Autodesk Inventor part; units mm, degrees
ref_plane "Work Plane5" through (-6.2, 0, 0) normal (-1, 0, 0) x (0, 0, 1)
ref_plane "YZ Plane" through (0, 0, 0) normal (1, 0, 0) x (0, 1, 0)
ref_plane "XZ Plane" through (0, 0, 0) normal (0, 1, 0) x (-1, 0, 0)
sketch "Sketch1" plane through (0, 0, 0) normal (0, 0, 1) x (1, 0, 0)
  line L0 (0, 0) -> (31, 0)
  line L1 (31, 0) -> (31, 4)
  line L2 (31, 4) -> (0, 4)
  line L3 (0, 4) -> (0, 0)
  line L4 (0, 18) -> (31, 18)
  line L5 (31, 18) -> (31, 20)
  line L6 (31, 20) -> (0, 20)
  line L7 (0, 20) -> (0, 18)
  line L8 (0, 34) -> (31, 34)
  line L9 (31, 34) -> (31, 38)
  line L10 (31, 38) -> (0, 38)
  line L11 (0, 38) -> (0, 34)
  line L12 (-7, 38) -> (0, 38)
  line L13 (0, 38) -> (0, 0)
  line L14 (0, 0) -> (-7, 0)
  line L15 (-7, 0) -> (-7, 38)
  line L16 (35, 38) -> (31, 38)
  line L17 (31, 38) -> (31, 0)
  line L18 (31, 0) -> (35, 0)
  line L19 (35, 0) -> (35, 38)
  point P0 (0, 4)
  point P1 (0, 18)
  point P2 (0, 20)
  point P3 (0, 34)
  dimension "d1" = 31
  dimension "d3" = 14
  dimension "d4" = 14
  dimension "d7" = 4
  dimension "d25" = 2
  dimension "d26" = 7
  dimension "d27" = 4
extrude "Extrusion1" add sketch "Sketch1" along normal blind 75 contours L3 L2 L1 L0 | L14 L15 L12 L11 L13 L7 L3 | L1 L17 L5 L9 L16 L19 L18 | L7 L6 L5 L4 | L10 L9 L8 L11
ref_plane "Work Plane5" through (-6.2, 0, 0) normal (-1, 0, 0) x (0, 0, 1)
sketch "Sketch4" plane through (-7, 0, 0) normal (-1, 0, 0) x (0, 0, 1)
  circle A0 centre (19, 19) radius 16.002
  circle A1 centre (56, 19) radius 16.002
  line L0 (75, 38) -> (75, 0)
  line L1 (0, 38) -> (0, 0)
  line L2 (56, 35.002) -> (72.002, 35.002)
  line L3 (72.002, 35.002) -> (72.002, 2.998)
  line L4 (72.002, 2.998) -> (56, 2.998)
  line L5 (19, 35.002) -> (35.002, 35.002)
  line L6 (35.002, 35.002) -> (35.002, 2.998)
  line L7 (35.002, 2.998) -> (19, 2.998)
  point P0 (0, 19)
  point P1 (35.002, 19)
  point P2 (72.002, 19)
  dimension "d28" = 32.004
  dimension "d29" = 32.004
  dimension "d32" = 19
  dimension "d33" = 19
extrude "Extrusion4" cut sketch "Sketch4" against normal blind 5.08 from surface at -0.8
fillet "Fillet2" radius 4 4 edges at (-7, 38, 37.5) (35, 38, 37.5) (35, 0, 37.5) (-7, 0, 37.5)
equation "\"d3\" = d4"
properties part number "Electronics Mount"
Read the model definition and answer for the solid it produces. Units are mm, in the model's axes. A direction names the side the tool comes from. Give positions to 0.01 mm unless a question says otherwise; leave off trailing zeros. Write each loop counter-clockwise with the first axis right and the second up, starting at its lowest first coordinate (ties: lowest second). Pieces come first, ordered by that corner, then holes. Notation, with made-up numbers: M 11,60 L 60,60 A25 cw 60,73 Z; hole C -33.5,-35.75 d2. An arc over 180 degrees is marked long. One line per item, written item: value. Start each with the question number.
(1) A tool of negligible diameter and unlimited length cuts with its end or side. For faces 1 (the flat face through (16, 4, 37)), 2 (the flat face through (-6.2, 19, 19)), 3 (the flat face through (14, 19, 75)), from which of +Z, -Z, +X, -X, +Y, -Y can it reach the whole face along a straight path? Write none if from no direction.
(2) Find section C-C (z = 20). Determine the outline of the cut face in (x, y), plus the area to 3 significant figures.
(3) Determine the mould class of faces 4 (the flat face through (-4, 19, 35.002)), 5 (the flat face through (-4, 35.002, 27)), 6 (the flat face through (14, 19, 0)), 7 (the cylindrical face through (-5.859, 1.203, 38.025)) for opening direction X: pulls with the +X half, pulls with the -X half, needs draft (parallel to the pull), parting line crosses it, or undercut.
(4) Flat-ended cylindrical pins translate along their axes: pin 1 Ø1.5 at (x, z) = (-5, 63) entering from -Y; pin 2 Ø1.5 at (x, z) = (-4, 26) entering from -Y. Find the tip coordinate at first contact, or state that the pin passes through.
(5) Find section A-A (x = 12). Determine the outline of the cut face in (y, z), plus the area to 3 significant figures.
(6) Find the intervals of material crossed by line 1 (X direction, y = 10, z = 14); line 2 (Y direction, x = 29, z = 45.5); line 3 (Z direction, x = -3, y = 23.5), in increasing order.
(7) Find section B-B (y = 7). Determine the outline of the cut face in (x, z).
(8) Find section D-D (y = 19). Determine the outline of the cut face in (x, z), plus the area to 3 significant figures.
Results below:
1. face 1: +Z, -Z
1. face 2: none
1. face 3: +Z, +X, -X, +Y, -Y
2. outline: M -7,4 A4 ccw -3,0 L 31,0 A4 ccw 35,4 L 35,34 A4 ccw 31,38 L -3,38 A4 ccw -7,34 Z; hole M -6.2,3 L -1.12,3 L -1.12,35 L -6.2,35 Z; hole M 0,4 L 31,4 L 31,18 L 0,18 Z; hole M 0,20 L 31,20 L 31,34 L 0,34 Z
2. area: 552 mm^2
3. face 4: undercut
3. face 5: undercut
3. face 6: needs draft
3. face 7: pulls with the -X half
4. pin 1: stops at y = 0.2
4. pin 2: stops at y = 0.01
5. outline: M 0,0 L 4,0 L 4,75 L 0,75 Z; M 18,0 L 20,0 L 20,75 L 18,75 Z; M 34,0 L 38,0 L 38,75 L 34,75 Z
5. area: 750 mm^2
6. line 1: x = -7 to -6.2, -1.12 to 0, 31 to 35
6. line 2: y = 0 to 4, 18 to 20, 34 to 38
6. line 3: z = 0 to 3.64, 35 to 40.64, 72 to 75
7. outline: M -7,0 L 0,0 L 0,75 L -7,75 Z; M 31,0 L 35,0 L 35,75 L 31,75 Z; hole M -6.2,8.41 L -1.12,8.41 L -1.12,35 L -6.2,35 Z; hole M -6.2,45.41 L -1.12,45.41 L -1.12,72 L -6.2,72 Z
8. outline: M -7,0 L 35,0 L 35,75 L -7,75 Z; hole M -6.2,3 L -1.12,3 L -1.12,35 L -6.2,35 Z; hole M -6.2,40 L -1.12,40 L -1.12,72 L -6.2,72 Z
8. area: 2,820 mm^2
